Verification items for the finished model (mm, model axes). A direction names the side the tool comes from. Give positions to 0.01 mm unless a question says otherwise; leave off trailing zeros. Write each loop counter-clockwise with the first axis right and the second up, starting at its lowest first coordinate (ties: lowest second). Pieces come first, ordered by that corner, then holes. Notation, with made-up numbers: (40, 79) -> (88, 79) arc R7 cw to (88, 86) -> close; hole circle Ø9 at (23, 52). An arc over 180 degrees is marked (long way). Use one line per item in the form item = value. Start each with the question number.
(1) Release check for a two-part mould opening along Y. For faces 1 (the face through (0, 0, 0)), 2 (the face through (0, -8.75, 4)), 3 (the face through (33.5, 0, 4)) record: pulls with the +Y half, pulls with the -Y half, needs draft (parallel to the pull), parting line crosses it, or undercut.
(2) Section check D-D, the plane z = 6.5. Record the cut outline in (x, y), plus the area to 3 significant figures.
(3) Section check A-A, the plane z = 3.25. Record the cut outline in (x, y), plus the area to 4 significant figures.
(4) Set-up check for faces 4 (the face through (33, 7, 4.5)), 5 (the face through (35, 0, 4)): record each of +Z, -Z, +X, -X, +Y, -Y from which the full face is reachable in a straight line by a thin tool's end or side.
(5) Scan lines: L1, parallel to X at y = 2.5, z = 5; L2, parallel to Y at x = -6.5, z = 6.25; L3, parallel to Z at x = -24, y = -1.75. Record each from-to range of solid material in increasing order.
(6) Depth check by flat-ended pin: pin 1 Ø1.7 at (x, y) = (-33.15, -6.9) entering from +Z; pin 2 Ø0.7 at (x, y) = (33.5, 7) entering from +Z; pin 3 Ø2 at (x, y) = (14, 2) entering from +Z. Enter the tip coordinate at first touch or a pass-through.
(7) Section check C-C, the plane x = 25.5. Record the cut outline in (y, z).
(8) Section check B-B, the plane y = 0. Record the cut outline in (x, z), plus the area to 3 significant figures.
from build123d import *

# Parameters (mm, degrees)
F0_W     = 70
F0_H     = 17.5
F1_DEPTH = 7.5
F2_T     = -1.5
F4_DEPTH = 6
F6_DEPTH = 3
F7_R     = 3.25
F8_DEPTH = 70.001


with BuildPart() as f1:
    # F0 (on Top) → F1 (new body)
    with BuildSketch(Plane.XY):
        Rectangle(F0_W, F0_H)
    extrude(amount=F1_DEPTH)

    # F2
    f2_openings = [f1.faces().sort_by_distance(p)[0] for p in [
        (0, 0, 7.5),
    ]]
    offset(amount=F2_T, openings=f2_openings)

    # F3 (on face) → F4 (join, through all)
    with BuildSketch(Plane.XY.offset(1.5)):
        Polygon((-33.5, 7.25), (-33.5, 4.421573), (-30.671573, 7.25), align=None)
        Polygon((30.671573, 7.25), (33.5, 4.421573), (33.5, 7.25), align=None)
        Polygon((33.5, -7.25), (33.5, -4.421573), (30.671573, -7.25), align=None)
        Polygon((-33.5, -4.421573), (-33.5, -7.25), (-30.671573, -7.25), align=None)
    extrude(amount=F4_DEPTH)

    # F5 (on face) → F6 (cut)
    with BuildSketch(Plane.XY.offset(7.5)):
        with BuildLine():
            ThreePointArc((-32.616117, 6.366117), (-32.453537, 6.609434), (-32.396447, 6.896447))
            ThreePointArc((-32.396447, 6.896447), (-33.839356, 7.183459), (-32.616117, 6.366117))
        make_face()
        with BuildLine():
            ThreePointArc((-32.616117, -6.366117), (-33.839356, -7.183459), (-32.396447, -6.896447))
            ThreePointArc((-32.396447, -6.896447), (-32.453537, -6.609434), (-32.616117, -6.366117))
        make_face()
        with BuildLine():
            ThreePointArc((32.616117, 6.366117), (33.433459, 6.203537), (33.896447, 6.896447))
            ThreePointArc((33.896447, 6.896447), (32.859434, 7.589356), (32.616117, 6.366117))
        make_face()
        with BuildLine():
            ThreePointArc((32.616117, -6.366117), (32.859434, -7.589356), (33.896447, -6.896447))
            ThreePointArc((33.896447, -6.896447), (33.433459, -6.203537), (32.616117, -6.366117))
        make_face()
    extrude(amount=-F6_DEPTH, mode=Mode.SUBTRACT)

    # F7 (on face) → F8 (cut, through all)
    with BuildSketch(Plane.YZ.offset(35)):
        with Locations((0, 7.5)):
            Circle(F7_R)
    extrude(amount=-F8_DEPTH, mode=Mode.SUBTRACT)


solid = f1.part
Completed:
q1.face_1 = needs draft
q1.face_2 = pulls with the -Y half
q1.face_3 = undercut
q2.outline = (-35, -8.75) -> (35, -8.75) -> (35, -3.09) -> (33.5, -3.09) -> (33.5, -4.42) -> (30.67, -7.25) -> (-30.67, -7.25) -> (-33.5, -4.42) -> (-33.5, -3.09) -> (-35, -3.09) -> close; (-35, 3.09) -> (-33.5, 3.09) -> (-33.5, 4.42) -> (-30.67, 7.25) -> (30.67, 7.25) -> (33.5, 4.42) -> (33.5, 3.09) -> (35, 3.09) -> (35, 8.75) -> (-35, 8.75) -> close; hole (-32.62, -6.37) arc R0.75 ccw (long way) to (-32.4, -6.9) arc R0.75 ccw to start; hole (-32.62, 6.37) arc R0.75 ccw to (-32.4, 6.9) arc R0.75 ccw (long way) to start; hole circle Ø1.5 at (33.15, -6.9); hole circle Ø1.5 at (33.15, 6.9)
q2.area = 244 mm²
q3.outline = (-35, -8.75) -> (35, -8.75) -> (35, 8.75) -> (-35, 8.75) -> close; hole (-33.5, -4.42) -> (-30.67, -7.25) -> (30.67, -7.25) -> (33.5, -4.42) -> (33.5, 4.42) -> (30.67, 7.25) -> (-30.67, 7.25) -> (-33.5, 4.42) -> close
q3.area = 269.5 mm²
q4.face_4 = +Z
q4.face_5 = +Z, -Z, +X, +Y, -Y
q5.L1 = -35 to -33.5, 33.5 to 35
q5.L2 = -8.75 to -7.25, 7.25 to 8.75
q5.L3 = 0 to 1.5
q6.pin_1 = 7.5
q6.pin_2 = 4.5
q6.pin_3 = 1.5
q7.outline = (-8.75, 0) -> (8.75, 0) -> (8.75, 7.5) -> (7.25, 7.5) -> (7.25, 1.5) -> (-7.25, 1.5) -> (-7.25, 7.5) -> (-8.75, 7.5) -> close
q8.outline = (-35, 0) -> (35, 0) -> (35, 4.25) -> (33.5, 4.25) -> (33.5, 1.5) -> (-33.5, 1.5) -> (-33.5, 4.25) -> (-35, 4.25) -> close
q8.area = 113 mm²
